from build123d import *

# Parameters (mm, degrees)
SKETCH1_W           = 5
SKETCH1_H           = 50
SKETCH1_W_2         = 70
SKETCH1_H_2         = 5
BOSS_EXTRUDE1_DEPTH = 50
SKETCH2_R           = 5
CUT_EXTRUDE1_DEPTH  = 5
FILLET1_R           = 10
FILLET2_R           = 12.5


with BuildPart() as part:
    # Sketch1 → Boss-Extrude1 (new body)
    with BuildSketch(Plane.XY):
        with Locations((2.5, -25)):
            Rectangle(SKETCH1_W, SKETCH1_H)
        with Locations((40, -52.5)):
            Rectangle(SKETCH1_W_2, SKETCH1_H_2)
        with Locations((2.5, -52.5)):
            Rectangle(SKETCH1_W, SKETCH1_H_2)
    extrude(amount=BOSS_EXTRUDE1_DEPTH)

    # Sketch2 → Cut-Extrude1 (cut)
    with BuildSketch(Plane.ZY):
        with Locations(Location((25, -25, 0), (0, 0, 270))):
            Circle(SKETCH2_R)
    extrude(amount=-CUT_EXTRUDE1_DEPTH, mode=Mode.SUBTRACT)

    # Fillet1
    fillet1_edges = [part.edges().sort_by_distance(p)[0] for p in [
        (0, -55, 25),
    ]]
    fillet(fillet1_edges, radius=FILLET1_R)

    # Fillet2
    fillet2_edges = [part.edges().sort_by_distance(p)[0] for p in [
        (2.5, 0, 50),
        (2.5, 0, 0),
    ]]
    fillet(fillet2_edges, radius=FILLET2_R)


solid = part.part
Geometry check sheet. Reference: the model listing, model coordinates, mm. A direction names the side the tool comes from. Round coordinates to 2 decimals unless told otherwise and drop trailing zeros. Order: outer loops, then holes, each group sorted by start corner. A loop starts at its lowest first (then second) coordinate and runs counter-clockwise, first axis right, second up. Notation, with made-up numbers: (69, 70) -> (115, 70) arc R30 ccw to (115, 108) -> close; hole circle Ø5 at (-11, -15). An arc over 180 degrees is marked (long way). Use one line per item in the form item = value.
1. Set-up check for faces 1 (the face through (26, -51, 0)), 2 (the face through (40, -50, 25)): record each of +Z, -Z, +X, -X, +Y, -Y from which the full face is reachable in a straight line by a thin tool's end or side.
Working result:
face_1 = -Z, +X, -X, +Y, -Y
face_2 = +Z, -Z, +X, +Y
2. Go/stop test with flat-tipped pins: pin 1 (16 mm diameter, centred on y = -25, z = 25, fed in from -X); pin 2 (25 mm diameter, centred on y = -29, z = 30.5, fed in from +X); pin 3 (3 mm diameter, centred on x = 55, z = 30, fed in from +Y). Record where each tip stops, or that it passes through.
Working result:
pin_1 = 0
pin_2 = 5
pin_3 = -50
3. Cross-section at B-B, the plane y = -25. Enter the section's corners in (x, z), plus the area to 3 significant figures.
Working result:
outline = (0, 0) -> (5, 0) -> (5, 20) -> (0, 20) -> close; (0, 30) -> (5, 30) -> (5, 50) -> (0, 50) -> close
area = 200 mm^2
4. Mould release check, pull along Y, two halves, no side actions. Record for faces 3 (the face through (2.85, -51.99, 25.35)), 4 (the face through (5, -31, 25)), 5 (the face through (2.46, -23.92, 20.12)), 6 (the face through (2, 0, 25)): pulls with the +Y half, pulls with the -Y half, needs draft (parallel to the pull), parting line crosses it, or undercut.
Working result:
face_3 = pulls with the -Y half
face_4 = needs draft
face_5 = undercut
face_6 = pulls with the +Y half
5. Cross-section at D-D, the plane x = 52. Enter the section's corners in (y, z), plus the area to 3 significant figures.
Working result:
outline = (-55, 0) -> (-50, 0) -> (-50, 50) -> (-55, 50) -> close
area = 250 mm^2
6. Scan lines: line 1 along Z through (x, y) = (3.5, -25); line 2 along X through (y, z) = (-39, 7); line 3 along Y through (x, z) = (11, 35.5). Record each from-to range of solid material in increasing order. Write a range as from..to.
Working result:
line_1 = 0..20, 30..50
line_2 = 0..5
line_3 = -55..-50
7. Cross-section at C-C, the plane z = 35.5. Enter the section's corners in (x, y), plus the area to 3 significant figures.
Working result:
outline = (0, -45) arc R10 ccw to (10, -55) -> (75, -55) -> (75, -50) -> (5, -50) -> (5, 0) -> (0, 0) -> close
area = 604 mm^2
8. Cross-section at A-A, the plane z = 25. Enter the section's corners in (x, y), plus the area to 3 significant figures.
Working result:
outline = (0, -45) arc R10 ccw to (10, -55) -> (75, -55) -> (75, -50) -> (5, -50) -> (5, -30) -> (0, -30) -> close; (0, -20) -> (5, -20) -> (5, 0) -> (0, 0) -> close
area = 554 mm^2
